Autodesk Inventor part; units mm, degrees
ref_plane "YZ Plane" through (0, 0, 0) normal (1, 0, 0) x (0, 1, 0)
ref_plane "XZ Plane" through (0, 0, 0) normal (0, 1, 0) x (-1, 0, 0)
ref_plane "XY Plane" through (0, 0, 0) normal (0, 0, 1) x (1, 0, 0)
sketch "Эскиз1" plane through (0, 0, 0) normal (0, 0, 1) x (1, 0, 0)
  line L0 (0, 8) -> (0, 15.15)
  line L1 (32.7, 15.15) -> (32.7, 15.15)
  line L2 (31.1, 13.55) -> (27.1142, 13.55)
  line L3 (26.4071, 13.8429) -> (25.1, 15.15)
  line L4 (25.1, 15.15) -> (0, 15.15)
  line L5 (-18, 0) -> (108, 0)
  arc A0 (31.1, 13.55) -> (32.7, 15.15) centre (31.1, 15.15) ccw
  arc A1 (26.4071, 13.8429) -> (27.1142, 13.55) centre (27.1142, 14.55) ccw
  line L6 (0, 8) -> (59.8, 8)
  line L7 (65.7, 21) -> (50, 21)
  line L8 (50, 21) -> (50, 26.5)
  line L9 (65.7, 21) -> (65.7, 21)
  line L10 (67.3, 19.4) -> (71.2858, 19.4)
  line L11 (71.9929, 19.6929) -> (73.3, 21)
  line L12 (73.3, 21) -> (90, 21)
  arc A2 (65.7, 21) -> (67.3, 19.4) centre (67.3, 21) ccw
  arc A3 (71.2858, 19.4) -> (71.9929, 19.6929) centre (71.2858, 20.4) ccw
  line L13 (32.7, 15.15) -> (32.7, 26.5)
  line L14 (32.7, 26.5) -> (50, 26.5)
  line L15 (59.8, 8) -> (59.8, 16.5)
  line L16 (59.8, 16.5) -> (59.8, 16.5)
  line L17 (61.4, 18.1) -> (65.3858, 18.1)
  line L18 (66.0929, 17.8071) -> (67.4, 16.5)
  line L19 (67.4, 16.5) -> (90, 16.5)
  line L20 (90, 16.5) -> (90, 21)
  arc A4 (66.0929, 17.8071) -> (65.3858, 18.1) centre (65.3858, 17.1) ccw
  arc A5 (61.4, 18.1) -> (59.8, 16.5) centre (61.4, 16.5) ccw
  point P0 (0, 0)
  point P1 (32.7, 13.55)
  point P2 (26.7, 13.55)
  point P3 (65.7, 19.4)
  point P4 (71.7, 19.4)
  point P5 (59.8, 18.1)
  point P6 (65.8, 18.1)
  dimension "d0" = 8
  dimension "d1" = 7.15
  dimension "d2" = 32.7
  dimension "d4" = 1.6
  dimension "d5" = 6
  dimension "d6" = 135
  dimension "d7" = 13.55
  dimension "d9" = 1.6
  dimension "d10" = 1
  dimension "d11" = 59.8
  dimension "d14" = 24.3
  dimension "d15" = 1.6
  dimension "d16" = 6
  dimension "d17" = 135
  dimension "d18" = 19.4
  dimension "d19" = 1.6
  dimension "d20" = 1
  dimension "d22" = 30.2
  dimension "d24" = 26.5
  dimension "d25" = 1.6
  dimension "d26" = 6
  dimension "d27" = 135
  dimension "d28" = 1
  dimension "d29" = 1.6
  dimension "d30" = 90
  dimension "d31" = 21
  dimension "d32" = 16.5
  dimension "d33" = 18.1
  dimension "d34" = 8
  dimension "d35" = 40
revolve "Вращение1" add sketch "Эскиз1" angle 360 about axis through (-10, 0, 0) along (1, 0, 0)
sketch "Эскиз2" plane through (0, 0, 0) normal (0, 1, 0) x (-1, 0, 0)
  line L0 (-32.7, 15.15) -> (-32.7, -15.15)
  line L1 (-32.7, 26.5) -> (-32.7, -26.5)
  line L2 (-32.7, 21.5) -> (-35.5868, 26.5)
  line L3 (-32.7, 21.5) -> (-26.9265, 21.5) construction
  line L4 (-32.7, 21.5) -> (-50, 21.5)
  line L5 (-50, 26.5) -> (-50, -26.5)
  line L6 (-50, 21.5) -> (-47.1132, 26.5)
  line L7 (-32.7, 26.5) -> (-50, 26.5)
  line L8 (-50, 21.5) -> (-44.2265, 21.5) construction
  line L9 (-47.1132, 26.5) -> (-50, 26.5)
  line L10 (-50, 26.5) -> (-50, 21.5)
  line L11 (-32.7, 21.5) -> (-32.7, 26.5)
  line L12 (-35.5868, 26.5) -> (-32.7, 26.5)
  line L13 (18, 0) -> (-108, 0)
  point P0 (0, 0)
  dimension "d38" = 120
  dimension "d39" = 60
  dimension "d45" = 21.5
  dimension "d46" = 26.5
  dimension "d47" = 2.8868
revolve "Вращение2" cut sketch "Эскиз2" angle 360 about axis through (-10, 0, 0) along (1, 0, 0) contours L2 L7 L1 | L5 L7 L6
sketch "Эскиз3" plane through (0, 0, 0) normal (1, 0, 0) x (0, 1, 0)
  line L0 (0, 26.5) -> (22.9497, 13.25)
  line L1 (22.9497, 13.25) -> (22.9497, -13.25)
  line L2 (22.9497, -13.25) -> (0, -26.5)
  line L3 (0, -26.5) -> (-22.9497, -13.25)
  line L4 (-22.9497, -13.25) -> (-22.9497, 13.25)
  line L5 (-22.9497, 13.25) -> (0, 26.5)
  line L6 (0, 34.2752) -> (29.6832, 17.1376)
  line L7 (29.6832, 17.1376) -> (29.6832, -17.1376)
  line L8 (29.6832, -17.1376) -> (0, -34.2752)
  line L9 (0, -34.2752) -> (-29.6832, -17.1376)
  line L10 (-29.6832, -17.1376) -> (-29.6832, 17.1376)
  line L11 (-29.6832, 17.1376) -> (0, 34.2752)
  point P0 (0, 0)
  point P1 (0, 0)
  point P2 (0, 0)
  point P3 (0, 0)
  dimension "d41" = 6.7335
  dimension "d42" = 52.6329
extrude "Выдавливание1" cut sketch "Эскиз3" along normal blind 271
chamfer "Фаска1" distance 2 angle 45 1 edges at (90, -21, 0)
chamfer "Фаска2" distance 1.5 angle 45 1 edges at (90, -16.5, 0)
chamfer "Фаска3" distance 2 angle 45 1 edges at (0, -15.15, 0)
chamfer "Фаска4" distance 1 angle 45 1 edges at (0, -8, 0)
thread "Резьба1"
thread "Резьба2"
thread "Резьба3"
properties part number "Штуцер"
Verification items for the finished model (mm, model axes). A direction names the side the tool comes from. Round coordinates to 2 decimals unless told otherwise and drop trailing zeros. Order: outer loops, then holes, each group sorted by start corner. A loop starts at its lowest first (then second) coordinate and runs counter-clockwise, first axis right, second up.
1. Thickness scan on L1, parallel to Z at x = 62, y = 0; L2, parallel to Z at x = 17, y = 0; L3, parallel to X at y = -15, z = 4.5. Record the ranges inside material, lowest first.
Final values:
L1: z = -21 to -18.1, 18.1 to 21
L2: z = -15.15 to -8, 8 to 15.15
L3: x = 32.7 to 59.8
2. Release check for a two-part mould opening along Y. For faces 1 (the flat face through (41.24, -11.31, -19.97)), 2 (the flat face through (59.8, -8, -3)), 3 (the conical face through (89.87, 8.83, 16.97)) record: +Y half, -Y half, draft (parallel to the pull), parting line (faces both ways), or undercut.
Final values:
face 1: -Y half
face 2: undercut
face 3: parting line
3. Access from +Z, -Z, +X, -X, +Y, -Y to the whole of each face (thin tool, end or side, straight path). Record for faces 4 (the cylindrical face through (30.81, -1.73, -7.81)), 5 (the cylindrical face through (69.321, 18.504, 5.827)), 6 (the cylindrical face through (57.74, 20.03, -6.31)).
Final values:
face 4: +X, -X
face 5: none
face 6: +X
4. Go/stop test with flat-tipped pins: P1, Ø4, axis at x = 51.5, y = -1, coming from the +Z side; P2, Ø13, axis at y = 0, z = 0, coming from the +X side; P3, Ø12, axis at x = 78.5, y = -6.5, coming from the +Z side; P4, Ø2, axis at y = 9.5, z = -3, coming from the +X side. Record where each tip stops, or that it passes through.
Final values:
P1: stops at z = 22.34
P2: passes through
P3: stops at z = 20.99
P4: stops at x = 59.8
5. Section check C-C on x = 29.5. Record the cut outline in (y, z), then the cut area to 3 significant figures.
Final values:
outline: circle Ø27.1 at (0, 0); hole circle Ø16 at (0, 0)
area: 376 mm2
6. Section check B-B on x = 80. Record the cut outline in (y, z), then the cut area to 3 significant figures.
Final values:
outline: circle Ø42 at (0, 0); hole circle Ø33 at (0, 0)
area: 530 mm2
